```python
from build123d import *

# Parameters (mm, degrees)
BASPROSKE_W         = 12.7
BASPROSKE_H         = 7.408333333
TOOTHCUT_DEPTH      = 17.463802889
TEETHCUTS_COUNT     = 12
TEETHCUTS_ANGLE     = 330
BORSKE_R            = 3.96875
BOSS_EXTRUDE1_DEPTH = 38.1
SKETCH2_W           = 4.30677954
SKETCH2_H           = 1.27
CUT_EXTRUDE1_DEPTH  = 2.54


with BuildPart() as part:
    # BasProSke → Base-Revolve (revolve)
    with BuildSketch(Plane(origin=(0, 0, 0), x_dir=(1, 0, 0), z_dir=(0, 1, 0)), mode=Mode.PRIVATE) as base_revolve_sk:
        with Locations((6.35, 3.704166667)):
            Rectangle(BASPROSKE_W, BASPROSKE_H)
    revolve(base_revolve_sk.sketch.rotate(Axis((-10, 0, 0), (1, 0, 0)), 180), axis=Axis((-10, 0, 0), (1, 0, 0)))

    # TooCutSke → ToothCut (cut, through all)
    with BuildSketch(Plane(origin=(0, 0, 0), x_dir=(0, 0, -1), z_dir=(1, 0, 0))):
        with BuildLine():
            ThreePointArc((0.598297521, 4.993485027), (0, 5.0292), (-0.598297521, 4.993485027))
            ThreePointArc((-0.598297521, 4.993485027), (-0.89092307, 6.262076537), (-1.773623584, 7.219047766))
            ThreePointArc((-1.773623584, 7.219047766), (0, 7.433733333), (1.773623584, 7.219047766))
            ThreePointArc((1.773623584, 7.219047766), (0.89092307, 6.262076537), (0.598297521, 4.993485027))
        make_face()
    toothcut = extrude(amount=TOOTHCUT_DEPTH, mode=Mode.SUBTRACT)

    # TeethCuts: ToothCut ×12 about axis
    teethcuts_axis = Axis((-10, 0, 0), (1, 0, 0))
    for i in range(1, TEETHCUTS_COUNT):
        add(toothcut.rotate(teethcuts_axis, i * TEETHCUTS_ANGLE / (TEETHCUTS_COUNT - 1)), mode=Mode.SUBTRACT)

    # BorSke → Boss-Extrude1 (add)
    with BuildSketch(Plane(origin=(0, 0, 0), x_dir=(0, 0, -1), z_dir=(1, 0, 0))):
        Circle(BORSKE_R)
    extrude(amount=-BOSS_EXTRUDE1_DEPTH)

    # Sketch2 → Cut-Extrude1 (cut)
    with BuildSketch(Plane.ZY.offset(38.1)):
        with Locations((0, 3.96875)):
            Rectangle(SKETCH2_W, SKETCH2_H)
    extrude(amount=-CUT_EXTRUDE1_DEPTH, mode=Mode.SUBTRACT)


solid = part.part
```
Model file for the job. Use its own axes, mm. Coordinates: 2 decimals unless noted, no trailing zeros. Loops run counter-clockwise (first coordinate to the right, second up) from the corner with the lowest first, then second, coordinate; pieces in that order, holes last. Notation, with made-up numbers: M -36.75,40 L 12.25,40 A20 ccw 12.25,56 Z; hole C 5.25,-2.75 d4. An arc over 180 degrees is marked long. Use CSV: the item, a comma, the result in double quotes. Start each with the question number.
1. Band-saw the part on D-D, the plane x = -11.5. List the corners of the cut face in (y, z).
2. Probe probe 1 along Z at (x, y) = (4.5, 4.5); probe 2 along Z at (x, y) = (-10.5, -0.25); probe 3 along X at (y, z) = (-3.5, -4.25). List the from-to ranges inside material, lowest first. Write a range as [from, to].
3. Flat gauge pins, fed straight in: pin 1 (1.5 mm diameter, centred on x = -15, z = -1.5, fed in from +Y); pin 2 (8 mm diameter, centred on x = -11, y = -1.5, fed in from +Z); pin 3 (1.3 mm diameter, centred on x = -37, z = 0.5, fed in from +Y). Where does each tip first touch, or does it go through?
4. Band-saw the part on C-C, the plane y = 0. List the corners of the cut face in (x, z), then the cut area to 3 significant figures.
5. Band-saw the part on B-B, the plane z = 0. List the corners of the cut face in (x, y).
6. Band-saw the part on A-A, the plane y = 6.25. List the corners of the cut face in (x, z), then the cut area to 3 significant figures.
7. Two-plate mould, pull along Y, no slides. Class faces 1 (the flat face through (-38.1, 0, 0)), 2 (the cylindrical face through (6.261, -3.903, -4.978)), 3 (the cylindrical face through (-18.783, -3.874, 0.86)): pulls with the +Y half, pulls with the -Y half, needs draft (parallel to the pull), parting line crosses it, or undercut.
Entries:
1,outline,"C 0,0 d7.94"
2,probe 1,"z = [-5.25, -3.34], [-2.25, 2.25], [3.34, 5.25]"
2,probe 2,"z = [-3.96, 3.96]"
2,probe 3,"x = [0, 12.7]"
3,pin 1,"stops at y = 3.9"
3,pin 2,"stops at z = 3.97"
3,pin 3,"stops at y = 3.33"
4,outline,"M -38.1,-3.97 L 0,-3.97 L 0,-5.03 L 12.7,-5.03 L 12.7,5.03 L 0,5.03 L 0,3.97 L -38.1,3.97 Z"
4,area,"430 mm2"
5,outline,"M -38.1,-3.97 L 0,-3.97 L 0,-5.03 L 12.7,-5.03 L 12.7,5.03 L 0,5.03 L 0,3.97 L -35.56,3.97 L -35.56,3.33 L -38.1,3.33 Z"
6,outline,"M 0,-2.35 L 12.7,-2.35 L 12.7,-0.88 L 0,-0.88 Z; M 0,0.88 L 12.7,0.88 L 12.7,2.35 L 0,2.35 Z"
6,area,"37.1 mm2"
7,face 1,"needs draft"
7,face 2,"undercut"
7,face 3,"parting line crosses it"
